from build123d import *

# Parameters (mm, degrees)
SKETCH1_R           = 2.4892
BOSS_EXTRUDE1_DEPTH = 3.175
FILLET1_R           = 4.7625


with BuildPart() as part:
    # Sketch1 → Boss-Extrude1 (new body)
    with BuildSketch(Plane(origin=(0, 0, 0), x_dir=(1, 0, 0), z_dir=(0, 1, 0))):
        Polygon((0, 25.4), (0, 0), (69.85, -40.64), (69.85, -50.8), (120.65, -50.8), (120.65, -40.64), (190.5, 0), (190.5, 25.4), align=None)
        Polygon((120.65, -33.293424872), (120.65, 0), (177.873073998, 0), align=None, mode=Mode.SUBTRACT)
        Polygon((69.85, -33.293424872), (12.626926002, 0), (69.85, 0), align=None, mode=Mode.SUBTRACT)
        with Locations((6.35, 12.7)):
            Circle(SKETCH1_R, mode=Mode.SUBTRACT)
        with Locations((31.75, 12.7)):
            Circle(SKETCH1_R, mode=Mode.SUBTRACT)
        with Locations((57.15, 12.7)):
            Circle(SKETCH1_R, mode=Mode.SUBTRACT)
        with Locations((82.55, 12.7)):
            Circle(SKETCH1_R, mode=Mode.SUBTRACT)
        with Locations((107.95, 12.7)):
            Circle(SKETCH1_R, mode=Mode.SUBTRACT)
        with Locations((133.35, 12.7)):
            Circle(SKETCH1_R, mode=Mode.SUBTRACT)
        with Locations((158.75, 12.7)):
            Circle(SKETCH1_R, mode=Mode.SUBTRACT)
        with Locations((184.15, 12.7)):
            Circle(SKETCH1_R, mode=Mode.SUBTRACT)
        with Locations((107.95, -6.35)):
            Circle(SKETCH1_R, mode=Mode.SUBTRACT)
        with Locations((82.55, -6.35)):
            Circle(SKETCH1_R, mode=Mode.SUBTRACT)
        with Locations((82.55, -44.45)):
            Circle(SKETCH1_R, mode=Mode.SUBTRACT)
        with Locations((82.55, -25.4)):
            Circle(SKETCH1_R, mode=Mode.SUBTRACT)
        with Locations((107.95, -44.45)):
            Circle(SKETCH1_R, mode=Mode.SUBTRACT)
        with Locations((107.95, -25.4)):
            Circle(SKETCH1_R, mode=Mode.SUBTRACT)
    extrude(amount=BOSS_EXTRUDE1_DEPTH)

    # Fillet1
    fillet1_edges = [part.edges().sort_by_distance(p)[0] for p in [
        (120.65, 1.5875, 33.293424872),
        (177.873073998, 1.5875, 0),
        (120.65, 1.5875, 0),
        (69.85, 1.5875, 33.293424872),
        (69.85, 1.5875, 0),
        (12.626926002, 1.5875, 0),
        (120.65, 1.5875, 40.64),
        (120.65, 1.5875, 50.8),
        (69.85, 1.5875, 50.8),
        (69.85, 1.5875, 40.64),
        (0, 1.5875, 0),
        (0, 1.5875, -25.4),
        (190.5, 1.5875, -25.4),
        (190.5, 1.5875, 0),
    ]]
    fillet(fillet1_edges, radius=FILLET1_R)


solid = part.part
Geometry check sheet. Reference: the model listing, model coordinates, mm. A direction names the side the tool comes from. Give positions to 0.01 mm unless a question says otherwise; leave off trailing zeros. Order: outer loops, then holes, each group sorted by start corner. A loop starts at its lowest first (then second) coordinate and runs counter-clockwise, first axis right, second up.
1) Material ranges on probe 1 along X at (y, z) = (1, 44.45); probe 2 along Z at (x, y) = (107.95, 2.35); probe 3 along X at (y, z) = (2.1, 42.5), recorded low to high.
Results are:
probe 1: x = 69.85 to 80.06, 85.04 to 105.46, 110.44 to 120.65
probe 2: z = -25.4 to -15.19, -10.21 to 3.86, 8.84 to 22.91, 27.89 to 41.96, 46.94 to 50.8
probe 3: x = 69.77 to 81, 84.1 to 106.4, 109.5 to 120.73
2) Cross-section at C-C (x = 140). Record the boundary of the cut face in (y, z) (3 decimals), then the cut area to 3 significant figures.
Results are:
outline: (0, -25.4) - (3.175, -25.4) - (3.175, 0) - (0, 0) - close; (0, 22.035) - (3.175, 22.035) - (3.175, 29.382) - (0, 29.382) - close
area: 104 mm2
3) Cross-section at D-D (y = 2.5). Give the number of separate pieces and of enclosed holes in the cut face, then the cut area to 3 significant figures.
Results are:
separate pieces: 1
enclosed holes: 16
area: 8,210 mm2
4) Draft check along X on faces 3 (the flat face through (94, 3.175, 4)), 4 (the cylindrical face through (0.62, 1.61, -0.39)), 5 (the cylindrical face through (82.01, 1.57, 27.83)). Enter one of: released by +X, released by -X, zero draft, split by the parting line, or undercut.
Results are:
face 3: zero draft
face 4: released by -X
face 5: undercut
5) Tool access check on faces 1 (the cylindrical face through (69.198, 1.61, 40.975)), 2 (the flat face through (145.454, 1.565, 18.862)). Record the directions out of +Z, -Z, +X, -X, +Y, -Y that give a thin tool (end or side, any length) a straight path to the whole face; none if there is none.
Results are:
face 1: +Z, -X, +Y, -Y
face 2: +Y, -Y
6) Gauge pin test, flat ends, axial feed: pin 1 (1.6 mm diameter, centred on x = 147.5, y = 1.5, fed in from +Z); pin 2 (1.3 mm diameter, centred on y = 1.5, z = 44, fed in from +X); pin 3 (1.6 mm diameter, centred on y = 2, z = 12, fed in from -X). Record the tip position at first contact, or that the pin passes through.
Results are:
pin 1: stops at z = 25.48
pin 2: stops at x = 120.65
pin 3: stops at x = 19.25
7) Cross-section at B-B (x = 57.15). Record the boundary of the cut face in (y, z) (3 decimals), then the cut area to 3 significant figures.
Results are:
outline: (0, -25.4) - (3.175, -25.4) - (3.175, -15.189) - (0, -15.189) - close; (0, -10.211) - (3.175, -10.211) - (3.175, 0) - (0, 0) - close; (0, 25.904) - (3.175, 25.904) - (3.175, 33.251) - (0, 33.251) - close
area: 88.2 mm2
8) Cross-section at A-A (z = 11.5). Record the boundary of the cut face in (x, y) (3 decimals).
Results are:
outline: (19.766, 0) - (32.393, 0) - (32.393, 3.175) - (19.766, 3.175) - close; (69.85, 0) - (120.65, 0) - (120.65, 3.175) - (69.85, 3.175) - close; (158.107, 0) - (170.734, 0) - (170.734, 3.175) - (158.107, 3.175) - close
